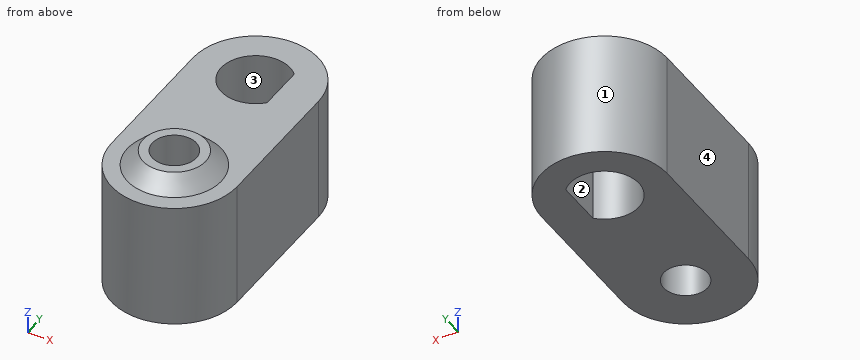
from build123d import *

# Parameters (mm, degrees)
EXTRUDE_2_DEPTH     = 8
SKETCH_1_6_R        = 1.4
CUT_EXTRUDE_2_DEPTH = 8
SKETCH_1_8_R        = 2
SKETCH_1_8_R_2      = 1.4
EXTRUDE_3_DEPTH     = 9
CHAMFER_2_SIZE      = 1


with BuildPart() as part:
    # 草图1 → 凸台-拉伸2 (new body)
    with BuildSketch(Plane.XY):
        with BuildLine():
            Line((4, 0), (4, -9))
            ThreePointArc((4, -9), (0, -13), (-4, -9))
            Line((-4, -9), (-4, 0))
            ThreePointArc((-4, 0), (0, 4), (4, 0))
        make_face()
    extrude(amount=EXTRUDE_2_DEPTH)

    # 草图1<6> → 切除-拉伸2 (cut)
    with BuildSketch(Plane.XY):
        with BuildLine():
            Line((1.6, -1.509966887), (1.6, 1.509966887))
            ThreePointArc((1.6, 1.509966887), (-2.2, 0), (1.6, -1.509966887))
        make_face()
        with Locations((0, -9)):
            Circle(SKETCH_1_6_R)
    extrude(amount=CUT_EXTRUDE_2_DEPTH, mode=Mode.SUBTRACT)

    # 草图1<8> → 凸台-拉伸3 (add)
    with BuildSketch(Plane.XY):
        with Locations((0, -9)):
            Circle(SKETCH_1_8_R)
        with Locations((0, -9)):
            Circle(SKETCH_1_8_R_2, mode=Mode.SUBTRACT)
    extrude(amount=EXTRUDE_3_DEPTH)

    # 倒角2
    chamfer_2_edges = [part.edges().sort_by_distance(p)[0] for p in [
        (-2, -9, 8),
    ]]
    chamfer(chamfer_2_edges, length=CHAMFER_2_SIZE - 0.0001)  # a hair under: the kernel refuses the full size


solid = part.part
Here's how the part is built. I have some questions about the finished solid (model axes, mm). Face numbers are marked on the shaded views. Round coordinates to 2 decimals unless told otherwise and drop trailing zeros. Order: outer loops, then holes, each group sorted by start corner. A loop starts at its lowest first (then second) coordinate and runs counter-clockwise, first axis right, second up. Notation, with made-up numbers: (-30, 29.5) -> (-25, 29.5) arc R36 cw to (-25, 64.5) -> close; hole circle Ø11 at (19.5, 48). An arc over 180 degrees is marked (long way). Return JSON: item names as keys, results as strings.
Q1. If we section it at B-B on z = 5.25: List the corners of the cut face in (x, y) for me, plus the area to 3 significant figures.
Filled sheet:
{"outline": "(-4, -9) arc R4 ccw to (4, -9) -> (4, 0) arc R4 ccw to (-4, 0) -> close; hole circle Ø2.8 at (0, -9); hole (1.6, -1.51) -> (1.6, 1.51) arc R2.2 ccw (long way) to start", "area": "102 mm^2"}
Q2. For pin 1 Ø1.5 at (x, y) = (2.5, 1.5) entering from +Z; pin 2 Ø2 at (x, y) = (0, -9) entering from +Z; pin 3 Ø1 at (x, z) = (-2.5, 1.5) entering from -Y, each with a flat end and sliding along its axis, tell me the tip position at first contact or that it passes through.
Filled sheet:
{"pin 1": "stops at z = 8", "pin 2": "passes through", "pin 3": "stops at y = -12.46"}
Q3. If we mould it in two halves opening along X, with no side actions, what happens to the marked faces 1, 2, 3 and 4? For each: released by +X, released by -X, zero draft, split by the parting line, or undercut.
Filled sheet:
{"face 1": "split by the parting line", "face 2": "undercut", "face 3": "undercut", "face 4": "released by -X"}
Q4. If we section it at C-C on y = -3: List the corners of the cut face in (x, z) for me, plus the area to 3 significant figures.
Filled sheet:
{"outline": "(-4, 0) -> (4, 0) -> (4, 8) -> (-4, 8) -> close", "area": "64.0 mm^2"}
Q5. I need wall thicknesses on line 1 along Y through (x, z) = (0, 2.5); line 2 along Z through (x, y) = (2.25, -7); line 3 along Y through (x, z) = (-1, 3.75). Which ranges of each line are inside material? Lowest first, please. Write a range as from..to.
Filled sheet:
{"line 1": "y = -13..-10.4, -7.6..-2.2, 2.2..4", "line 2": "z = 0..8", "line 3": "y = -12.87..-9.98, -8.02..-1.96, 1.96..3.87"}
Q6. If we section it at A-A on x = 0: Give the number of separate pieces and of enclosed holes in the cut face, plus the area to 3 significant figures.
Filled sheet:
{"separate pieces": "3", "enclosed holes": "0", "area": "80.6 mm^2"}
